Check sheet for the drawn part. Datum: minimum x, y, z corner. Units: mm. A direction names the side the tool comes from. Coordinates: 2 decimals unless noted, no trailing zeros. Order: outer loops, then holes, each group sorted by start corner. A loop starts at its lowest first (then second) coordinate and runs counter-clockwise, first axis right, second up. Notation, with made-up numbers: (29.5, 88.25) -> (77.5, 88.25) arc R14 ccw to (77.5, 114.25) -> close; hole circle Ø8 at (47.25, 72.5). An arc over 180 degrees is marked (long way). Answer as CSV lines item,"result".
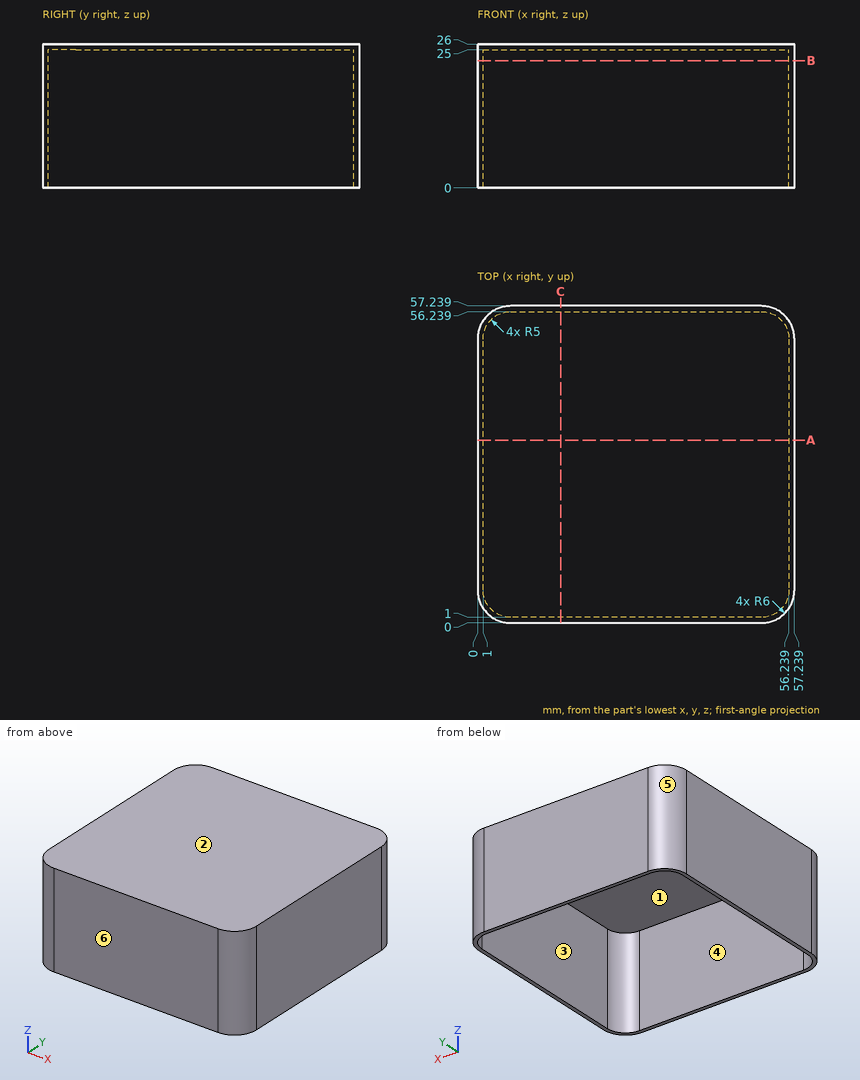
Item 1: Depth check by flat-ended pin: pin 1 Ø3 at (x, y) = (12, 33.5) entering from -Z. Enter the tip coordinate at first touch or a pass-through.
Answer list:
pin 1,"z = 25"
Item 2: Release check for a two-part mould opening along Y. For the marked faces 3, 4, 5 and 6 record: +Y half, -Y half, draft (parallel to the pull), parting line (faces both ways), or undercut.
Answer list:
face 3,"undercut"
face 4,"undercut"
face 5,"+Y half"
face 6,"-Y half"
Item 3: Tool access check on the marked faces 1 and 2. Record the directions out of +Z, -Z, +X, -X, +Y, -Y that give a thin tool (end or side, any length) a straight path to the whole face; none if there is none.
Answer list:
face 1,"-Z"
face 2,"+Z, +X, -X, +Y, -Y"
Item 4: Section check A-A, the plane y = 33. Record the boundary of the cut face in (x, z).
Answer list:
outline,"(0, 0) -> (1, 0) -> (1, 25) -> (56.24, 25) -> (56.24, 0) -> (57.24, 0) -> (57.24, 26) -> (0, 26) -> close"
Item 5: Thickness scan on line 1 (X direction, y = 28.5, z = 10.75); line 2 (Z direction, x = 18, y = 45). Record the ranges inside material, lowest first.
Answer list:
line 1,"0 to 1, 56.24 to 57.24"
line 2,"25 to 26"
Item 6: Section check B-B, the plane z = 23. Record the boundary of the cut face in (x, y).
Answer list:
outline,"(0, 6) arc R6 ccw to (6, 0) -> (51.24, 0) arc R6 ccw to (57.24, 6) -> (57.24, 51.24) arc R6 ccw to (51.24, 57.24) -> (6, 57.24) arc R6 ccw to (0, 51.24) -> close; hole (1, 6) arc R5 ccw to (6, 1) -> (51.24, 1) arc R5 ccw to (56.24, 6) -> (56.24, 51.24) arc R5 ccw to (51.24, 56.24) -> (6, 56.24) arc R5 ccw to (1, 51.24) -> close"
